Geometry: final body of the model. Coordinates: model frame, mm. Face numbers are marked on the shaded views. Give positions to 0.01 mm unless a question says otherwise; leave off trailing zeros. Order: outer loops, then holes, each group sorted by start corner. A loop starts at its lowest first (then second) coordinate and runs counter-clockwise, first axis right, second up. Notation, with made-up numbers: (38, -29.5) - (93, -29.5) arc R9 cw to (93, -20.5) - close; hole circle Ø3 at (18, 22.5). An arc over 180 degrees is marked (long way). Use one line per item in the form item = value.
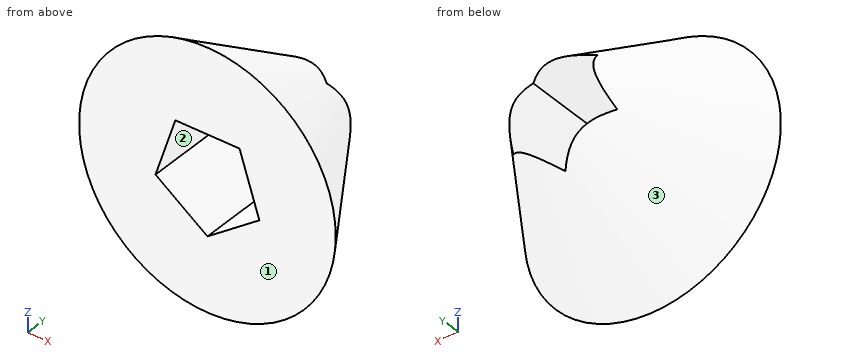
Autodesk Inventor part; units mm, degrees
ref_plane "YZ Plane" through (0, 0, 0) normal (1, 0, 0) x (0, 1, 0)
ref_plane "XZ Plane" through (0, 0, 0) normal (0, 1, 0) x (-1, 0, 0)
ref_plane "XY Plane" through (0, 0, 0) normal (0, 0, 1) x (1, 0, 0)
sketch "Эскиз1" plane through (0, 0, 0) normal (0, 0, 1) x (1, 0, 0)
  line L0 (0, 0) -> (10, 0)
  line L1 (10, 0) -> (0, 15.3986)
  line L2 (0, 15.3986) -> (0, 0)
  dimension "d0" = 10
  dimension "d1" = 57
revolve "Вращение1" add sketch "Эскиз1" angle 360 about axis through (0, 15.3986, 0) along (0, -1, 0)
sketch "Эскиз2" plane through (0, 0, 0) normal (0, 1, 0) x (-1, 0, 0)
  line L0 (0, -4.2533) -> (-4.0451, -1.3143)
  line L1 (-4.0451, -1.3143) -> (-2.5, 3.441)
  line L2 (-2.5, 3.441) -> (2.5, 3.441)
  line L3 (2.5, 3.441) -> (4.0451, -1.3143)
  line L4 (4.0451, -1.3143) -> (0, -4.2533)
  point P0 (0, 0)
  point P1 (0, 0)
  dimension "d3" = 5
extrude "Выдавливание1" cut sketch "Эскиз2" along normal blind 40
properties part number "1"
(1) Cut plane A-A on z = 0. Output: boundary loops of the cut face in (x, y).
Computed values:
outline = (-10, 0) - (-3.62, 0) - (-3.62, 9.83) - close; (3.62, 0) - (10, 0) - (3.62, 9.83) - close
(2) Contact query for flat-ended pins moving along their axis: pin 1 Ø5.5 at (x, y) = (0.5, 6.5) entering from -Z; pin 2 Ø1 at (x, y) = (4.5, 7.5) entering from +Z; pin 3 Ø1 at (y, z) = (1.5, 7) entering from +X. Output: stop coordinate, or through.
Computed values:
pin_1 = -7.55
pin_2 = 3.4
pin_3 = 6.44
(3) Ray query, line 1 along Z through (x, y) = (1.75, 1); line 2 along Z through (x, y) = (0.25, 3); line 3 along X through (y, z) = (4.25, -0.5). Return the intervals inside material, ascending.
Computed values:
line_1 = -9.19 to -2.98, 3.44 to 9.19
line_2 = -8.05 to -4.07, 3.44 to 8.05
line_3 = -7.22 to -3.78, 3.78 to 7.22
(4) Cut plane B-B on y = 2. Output: boundary loops of the cut face in (x, z).
Computed values:
outline = circle Ø17.4 at (0, 0); hole (-4.05, -1.31) - (0, -4.25) - (4.05, -1.31) - (2.5, 3.44) - (-2.5, 3.44) - close
(5) Pull-direction query (Z, two-part tool) for the marked faces 1, 2 and 3; classes: released by +Z, released by -Z, zero draft, split by the parting line, or undercut.
Computed values:
face_1 = zero draft
face_2 = undercut
face_3 = split by the parting line
(6) Cut plane C-C on y = 4.5. Output: boundary loops of the cut face in (x, z), plus the area to 3 significant figures.
Computed values:
outline = circle Ø14.16 at (0, 0); hole (-4.05, -1.31) - (0, -4.25) - (4.05, -1.31) - (2.5, 3.44) - (-2.5, 3.44) - close
area = 114 mm²
